Design review of the part shown in the three views and the two pictorial views. Dimensions are in mm from the part's minimum x, y and z. A direction names the side the tool comes from. Give positions to 0.01 mm unless a question says otherwise; leave off trailing zeros. Loops run counter-clockwise (first coordinate to the right, second up) from the corner with the lowest first, then second, coordinate; pieces in that order, holes last. Notation, with made-up numbers: (20, -29.75) -> (48, -29.75) arc R16 ccw to (48, -9.75) -> close; hole circle Ø5 at (16.5, 72.5). An arc over 180 degrees is marked (long way). Use CSV: the item, a comma, the result in double quotes. Start each with the question number.
Item 1: Clearance check with flat-ended pins moving along their axes: pin 1 (6.5 mm diameter, centred on x = 4, y = 9, fed in from +Z); pin 2 (9 mm diameter, centred on y = 8.5, z = 13.5, fed in from -X); pin 3 (1.5 mm diameter, centred on y = 3.5, z = 5.5, fed in from +X); pin 4 (2 mm diameter, centred on y = 2.5, z = 11, fed in from -X). State where each tip first meets the part, or that it passes through.
Item 2: We need section D-D (y = 11.75). State the section outline as (x, z) points.
Item 3: For the marked faces 5, 6 and 7, list the 3-axis set-ups (+Z, -Z, +X, -X, +Y, -Y) from which the entire face can be reached by the end or side of a thin tool; tool diameter is ignored.
Item 4: We need section C-C (x = 4). State the section outline as (y, z) points.
Item 5: Wall thickness on line 1 along Y through (x, z) = (14.25, 1); line 2 along X through (y, z) = (6.25, 4.5); line 3 along X through (y, z) = (6, 10): over which ranges is each line inside the solid? List them lowest first. Write a range as from..to.
Item 6: We need section B-B (z = 10.75). State the section outline as (x, y) points.
Item 7: We need section A-A (y = 9). State the section outline as (x, z) points, plus the area to 3 significant figures.
Item 8: The part is to be moulded in two halves that separate along Y. For the marked faces 1, 2, 3 and 4, say which applies: +Y half, -Y half, draft (parallel to the pull), parting line (faces both ways), or undercut.
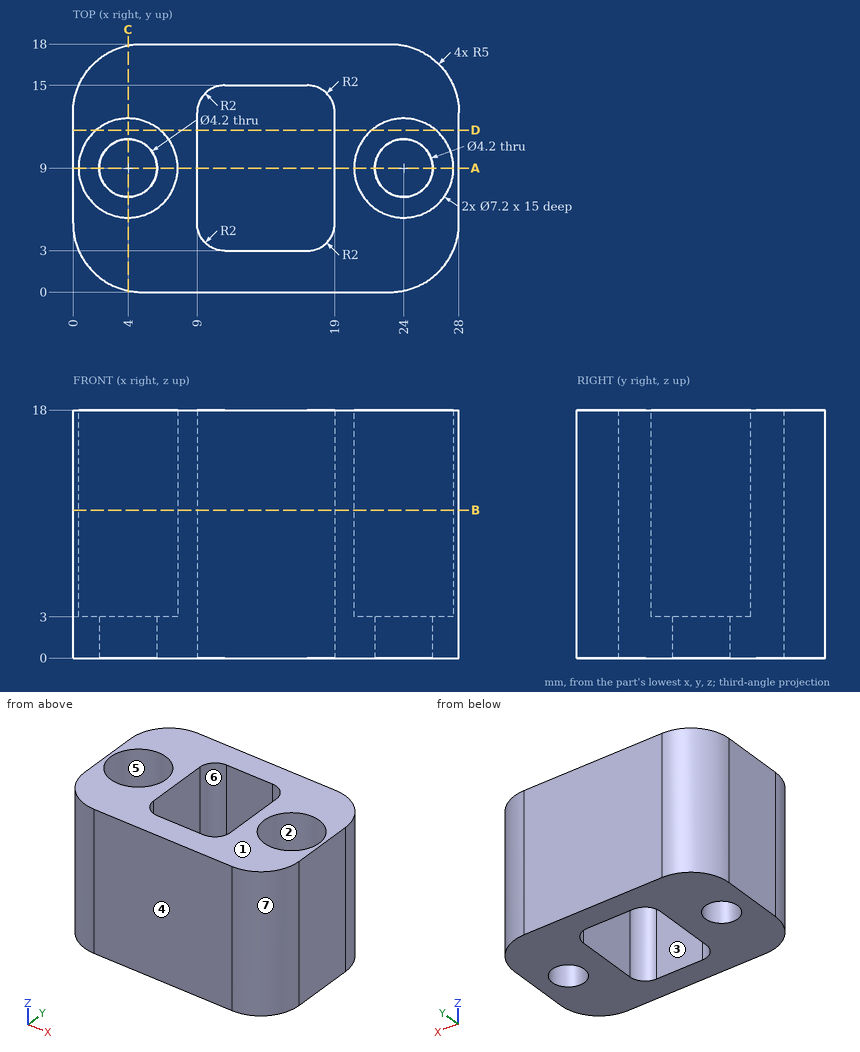
Results found:
1,pin 1,"z = 3"
1,pin 2,"x = 0"
1,pin 3,"x = 27.94"
1,pin 4,"x = 0.23"
2,outline,"(0, 0) -> (9, 0) -> (9, 18) -> (6.32, 18) -> (6.32, 3) -> (1.68, 3) -> (1.68, 18) -> (0, 18) -> close; (19, 0) -> (28, 0) -> (28, 18) -> (26.32, 18) -> (26.32, 3) -> (21.68, 3) -> (21.68, 18) -> (19, 18) -> close"
3,face 5,"+Z"
3,face 6,"+Z, -Z"
3,face 7,"+Z, -Z, +X, -Y"
4,outline,"(0.1, 0) -> (6.9, 0) -> (6.9, 3) -> (5.4, 3) -> (5.4, 18) -> (0.1, 18) -> close; (11.1, 0) -> (17.9, 0) -> (17.9, 18) -> (12.6, 18) -> (12.6, 3) -> (11.1, 3) -> close"
5,line 1,"0..3, 15..18"
5,line 2,"0..1.68, 6.32..9, 19..21.68, 26.32..28"
5,line 3,"0..2.01, 5.99..9, 19..22.01, 25.99..28"
6,outline,"(0, 5) arc R5 ccw to (5, 0) -> (23, 0) arc R5 ccw to (28, 5) -> (28, 13) arc R5 ccw to (23, 18) -> (5, 18) arc R5 ccw to (0, 13) -> close; hole circle Ø7.2 at (4, 9); hole (9, 5) arc R2 ccw to (11, 3) -> (17, 3) arc R2 ccw to (19, 5) -> (19, 13) arc R2 ccw to (17, 15) -> (11, 15) arc R2 ccw to (9, 13) -> close; hole circle Ø7.2 at (24, 9)"
7,outline,"(0, 0) -> (1.9, 0) -> (1.9, 3) -> (0.4, 3) -> (0.4, 18) -> (0, 18) -> close; (6.1, 0) -> (9, 0) -> (9, 18) -> (7.6, 18) -> (7.6, 3) -> (6.1, 3) -> close; (19, 0) -> (21.9, 0) -> (21.9, 3) -> (20.4, 3) -> (20.4, 18) -> (19, 18) -> close; (26.1, 0) -> (28, 0) -> (28, 18) -> (27.6, 18) -> (27.6, 3) -> (26.1, 3) -> close"
7,area,"82.8 mm²"
8,face 1,"draft"
8,face 2,"undercut"
8,face 3,"undercut"
8,face 4,"-Y half"
